Input: dimensioned drawing with shaded views. Units: mm. Origin: part minimum x, y, z. A direction names the side the tool comes from. Round coordinates to 2 decimals unless told otherwise and drop trailing zeros. Loops run counter-clockwise (first coordinate to the right, second up) from the corner with the lowest first, then second, coordinate; pieces in that order, holes last. Notation, with made-up numbers: M -18,56 L -5,56 A14 ccw -5,60 Z; hole C 9.5,7.5 d9. An arc over 180 degrees is marked long. Put each result on its own line as item: value. Start each with the question number.
1) Section A-A on y = 33. Output: boundary loops of the cut face in (x, z) (1 decimal).
2) Reachability of the marked faces 1, 2 and 3 from +Z, -Z, +X, -X, +Y, -Y: full face, straight path, thin tool, end or side. Return the list, or none.
3) Line query: probe 1 along X at (y, z) = (233.5, 75.5); probe 2 along Z at (x, y) = (58.5, 225.5) (1 decimal); probe 3 along Y at (x, z) = (85, 131). Output: solid intervals per line, ascending.
4) Pin query (flat end, axial travel): pin 1 (1 mm diameter, centred on y = 119, z = 121.5, fed in from +X); pin 2 (10 mm diameter, centred on x = 83, z = 96.5, fed in from -Y); pin 3 (6 mm diameter, centred on x = 108.5, y = 205.5, fed in from -Z). Return the tip coordinate at first contact, or that it passes through.
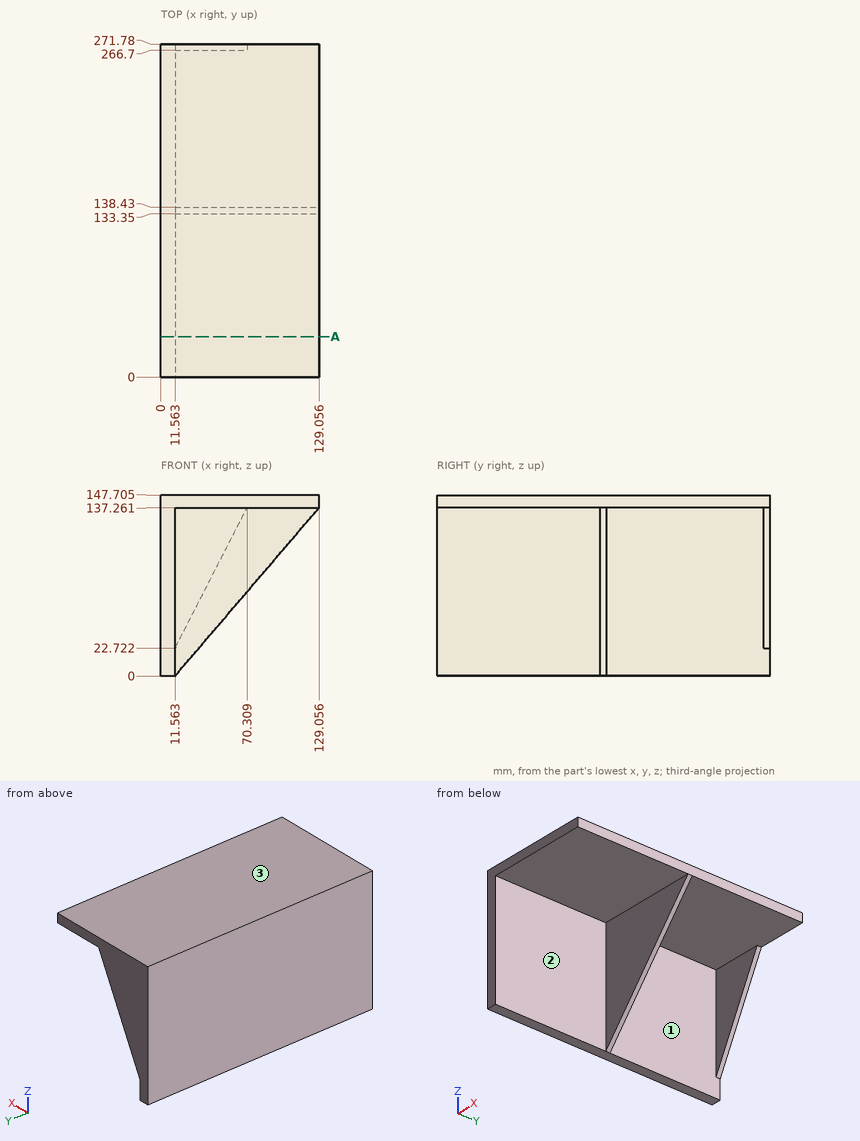
Geometry results:
1. outline: M 0,0 L 11.6,0 L 11.6,137.3 L 129.1,137.3 L 129.1,147.7 L 0,147.7 Z
2. face 1: -Z, +X
2. face 2: -Z, +X, -Y
2. face 3: +Z, +X, -X, +Y, -Y
3. probe 1: x = 0 to 11.56
3. probe 2: z = 137.3 to 147.7
3. probe 3: y = 133.35 to 138.43
4. pin 1: stops at x = 11.56
4. pin 2: stops at y = 133.35
4. pin 3: stops at z = 137.26
